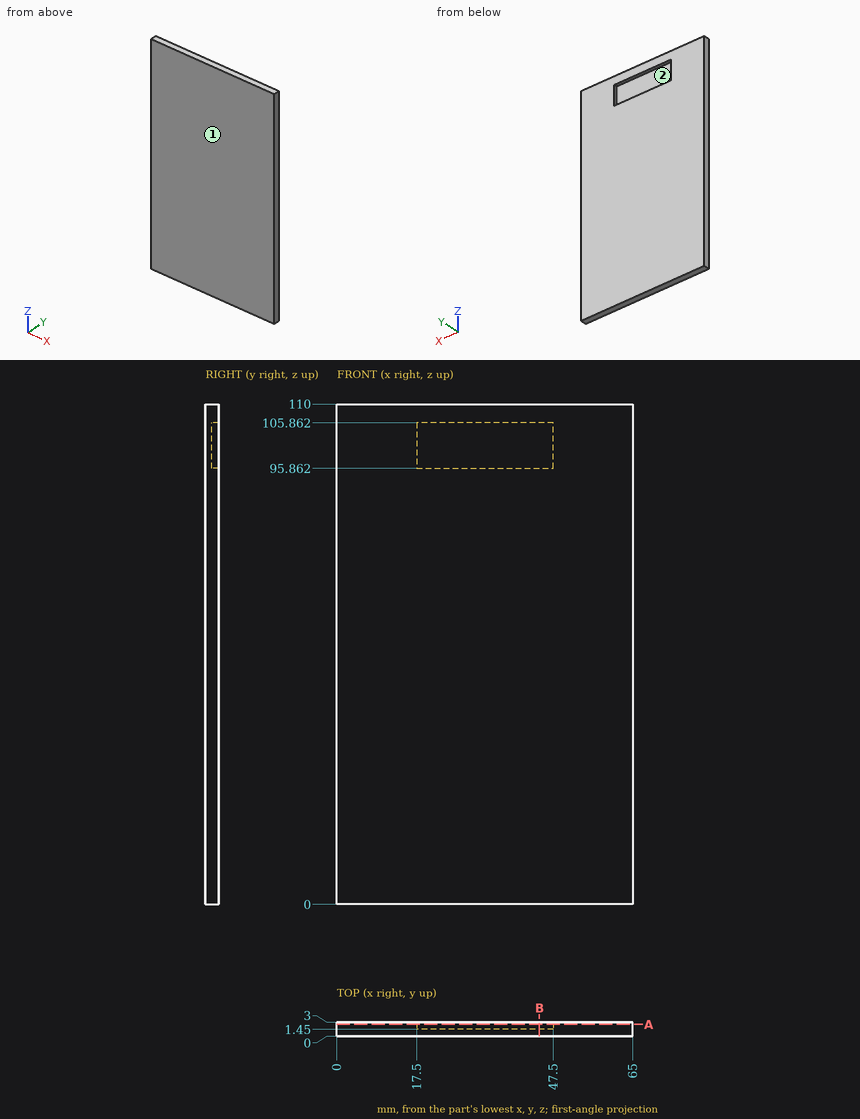
Here's the drawing with two shaded views (mm, measured from the low corner). I have some questions. Round coordinates to 2 decimals unless told otherwise and drop trailing zeros. Write each loop counter-clockwise with the first axis right and the second up, starting at its lowest first coordinate (ties: lowest second). Pieces come first, ordered by that corner, then holes. Notation, with made-up numbers: M 12,-26.75 L 46,-26.75 A24 ccw 46,4.25 Z; hole C 62,74.5 d10. An arc over 180 degrees is marked long. Answer in a Markdown table with one row per item. Add a question column.
Q1. Imagine slicing it at B-B (x = 44.5). Please give me the cut outline in (y, z).
Q2. If I drill on line 1 (Z direction, x = 37.5, y = 2); line 2 (Y direction, x = 44, z = 96), over which ranges is the centre line in solid material (lowest first)? Write a range as from..to.
Q3. If we mould it in two halves opening along X, with no side actions, what happens to the marked faces 1 and 2? For each: +X half, -X half, draft (parallel to the pull), parting line (faces both ways), or undercut.
Q4. Will this pin go through, and if not, where does the flat tip stop? pin 1 Ø8 at (x, z) = (31, 101.5) entering from +Y.
Q5. Imagine slicing it at A-A (y = 2.55). Please give me the cut outline in (x, z), then the cut area to 3 significant figures.
Values:
| question | item | result |
|---|---|---|
| 1 | outline | M 0,0 L 3,0 L 3,95.86 L 1.45,95.86 L 1.45,105.86 L 3,105.86 L 3,110 L 0,110 Z |
| 2 | line 1 | 0..95.86, 105.86..110 |
| 2 | line 2 | 0..1.45 |
| 3 | face 1 | draft |
| 3 | face 2 | undercut |
| 4 | pin 1 | y = 1.45 |
| 5 | outline | M 0,0 L 65,0 L 65,110 L 0,110 Z; hole M 17.5,95.86 L 47.5,95.86 L 47.5,105.86 L 17.5,105.86 Z |
| 5 | area | 6,850 mm^2 |
